```python
from build123d import *

# Parameters (mm, degrees)
BOSS_EXTRU_1_DEPTH           = 300
ENL_V_MAT_EXTRU_1_DEPTH      = 305.05591591
ENL_V_MAT_EXTRU_1_DEPTH_BACK = 305.05591591
ESQUISSE2_R                  = 2.5
ENL_V_MAT_EXTRU_2_DEPTH      = 305.1397705
ENL_V_MAT_EXTRU_2_DEPTH_BACK = 305.1397705
ESQUISSE3_R                  = 1.65


with BuildPart() as part:
    # Esquisse1 → Boss.-Extru.1 (new body)
    with BuildSketch(Plane.XY):
        Polygon((0, 0), (0, 10), (8, 10), (8, 3), (41, 3), (41, 10), (49, 10), (49, 0), align=None)
    extrude(amount=BOSS_EXTRU_1_DEPTH)

    # Esquisse2 → Enlèv. mat.-Extru.1 (cut, two sides: drawn at the far end of the back side and taken through both)
    with BuildSketch(Plane(origin=(0, 3, 0), x_dir=(1, 0, 0), z_dir=(0, 1, 0)).offset(-ENL_V_MAT_EXTRU_1_DEPTH_BACK)):
        with Locations(Location((17.5, -120, 0), (0, 0, 270))):
            Circle(ESQUISSE2_R)
        with Locations(Location((31.5, -120, 0), (0, 0, 90))):
            Circle(ESQUISSE2_R)
    extrude(amount=ENL_V_MAT_EXTRU_1_DEPTH + ENL_V_MAT_EXTRU_1_DEPTH_BACK, mode=Mode.SUBTRACT)

    # Esquisse3 → Enlèv. mat.-Extru.2 (cut, two sides: drawn at the far end of the back side and taken through both)
    with BuildSketch(Plane(origin=(0, 10, 0), x_dir=(1, 0, 0), z_dir=(0, 1, 0)).offset(-ENL_V_MAT_EXTRU_2_DEPTH_BACK)):
        with Locations(Location((45, -270, 0), (0, 0, 270))):
            Circle(ESQUISSE3_R)
        with Locations(Location((45, -190, 0), (0, 0, 270))):
            Circle(ESQUISSE3_R)
        with Locations(Location((45, -110, 0), (0, 0, 90))):
            Circle(ESQUISSE3_R)
        with Locations(Location((45, -30, 0), (0, 0, 90))):
            Circle(ESQUISSE3_R)
        with Locations(Location((4, -30, 0), (0, 0, 270))):
            Circle(ESQUISSE3_R)
        with Locations(Location((4, -110, 0), (0, 0, 270))):
            Circle(ESQUISSE3_R)
        with Locations(Location((4, -190, 0), (0, 0, 90))):
            Circle(ESQUISSE3_R)
        with Locations(Location((4, -270, 0), (0, 0, 90))):
            Circle(ESQUISSE3_R)
    extrude(amount=ENL_V_MAT_EXTRU_2_DEPTH + ENL_V_MAT_EXTRU_2_DEPTH_BACK, mode=Mode.SUBTRACT)


solid = part.part
```
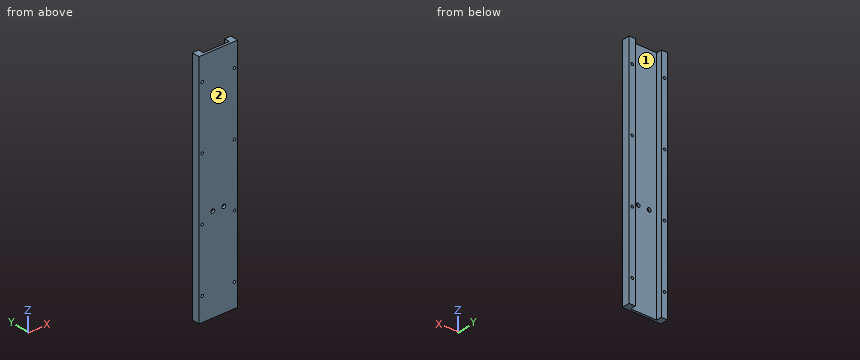
For this review, take the finished solid that the model builds, in its own axes (mm). Face numbers are marked on the shaded views. Round coordinates to 2 decimals unless told otherwise and drop trailing zeros. Write each loop counter-clockwise with the first axis right and the second up, starting at its lowest first coordinate (ties: lowest second). Pieces come first, ordered by that corner, then holes. Notation, with made-up numbers: M 55,70 L 75,70 A15 cw 75,99 Z; hole C -39,1.25 d11. An arc over 180 degrees is marked long. One line per item, written item: value. Start each with the question number.
(1) We need section A-A (y = 6). Count the separate pieces of the cut face and the enclosed holes in it, and give its area (3 significant figures).
(2) Insertion check: pin 1 (2 mm diameter, centred on x = 4, z = 110, fed in from +Y); pin 2 (16.5 mm diameter, centred on x = 32, z = 82, fed in from +Y); pin 3 (5.5 mm diameter, centred on x = 4, z = 190, fed in from -Y). Each pin has a flat end and moves straight along its axis. Give the tip position at first contact, or say it passes through.
(3) We need section B-B (x = 17.5). Give the boundary of the cut face in (y, z).
(4) The part is to be moulded in two halves that separate along X. For the marked faces 1 and 2, say which applies: released by +X, released by -X, zero draft, split by the parting line, or undercut.
(5) We need section C-C (z = 238). Give the boundary of the cut face in (x, y), and give its area (3 significant figures).
(6) Wall thickness on line 1 (X direction, y = 2.1, z = 120); line 2 (X direction, y = 2, z = 190); line 3 (X direction, y = 4.5, z = 236): over which ranges is each line inside the solid? List them lowest first.
Result:
1. separate pieces: 2
1. enclosed holes: 8
1. area: 4,730 mm²
2. pin 1: through
2. pin 2: y = 3
2. pin 3: y = 0
3. outline: M 0,0 L 3,0 L 3,117.5 L 0,117.5 Z; M 0,122.5 L 3,122.5 L 3,300 L 0,300 Z
4. face 1: undercut
4. face 2: zero draft
5. outline: M 0,0 L 49,0 L 49,10 L 41,10 L 41,3 L 8,3 L 8,10 L 0,10 Z
5. area: 259 mm²
6. line 1: 0 to 15, 20 to 29, 34 to 49
6. line 2: 0 to 2.35, 5.65 to 43.35, 46.65 to 49
6. line 3: 0 to 8, 41 to 49
